Verification items for the finished model (mm, model axes). Coordinates: 2 decimals unless noted, no trailing zeros. Order: outer loops, then holes, each group sorted by start corner. A loop starts at its lowest first (then second) coordinate and runs counter-clockwise, first axis right, second up. Notation, with made-up numbers: (68.5, -34) -> (96.5, -34) arc R33 ccw to (96.5, 1) -> close; hole circle Ø11 at (69, 88). An arc over 180 degrees is marked (long way). Write item = value, one per line. Start each with the question number.
1. Cross-section at C-C on x = 13.5. Record the cut outline in (y, z), plus the area to 3 significant figures.
2. Thickness scan on line 1 along Z through (x, y) = (5.5, 20.5); line 2 along X through (y, z) = (21.25, -4); line 3 along Z through (x, y) = (-8.5, 21.5). Record the ranges inside material, lowest first. Write a range as from..to.
3. Cross-section at A-A on y = 23. Record the cut outline in (x, z), plus the area to 3 significant figures.
4. Go/stop test with flat-tipped pins: P1, Ø4, axis at x = 8.5, z = 1, coming from the -Y side; P2, Ø8, axis at x = 2.5, z = -8, coming from the -Y side; P3, Ø3, axis at x = -12, z = 6, coming from the +Y side. Record where each tip stops, or that it passes through.
5. Cross-section at B-B on z = -2. Record the cut outline in (x, y).
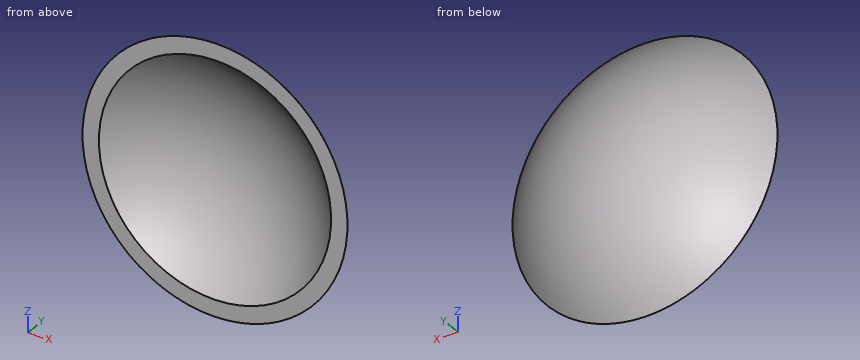
from build123d import *

# Parameters (mm, degrees)
BOX_W           = 60
BOX_H           = 60
BOX_DEPTH       = 60
SPHERE001_ANGLE = 180
SPHERE_ANGLE    = 180


with BuildPart() as cube:
    # Box → Box (new body)
    with BuildSketch(Plane(origin=(-30, -40, -30), x_dir=(1, 0, 0), z_dir=(0, 0, 1))):
        with Locations((30, 30)):
            Rectangle(BOX_W, BOX_H)
    extrude(amount=BOX_DEPTH)


with BuildPart() as inner:
    # Sphere001 → Sphere001 (revolve)
    with BuildSketch(Plane.XZ):
        with BuildLine():
            ThreePointArc((0, -28), (28, 0), (0, 28))
            Line((0, 28), (0, -28))
        make_face()
    revolve(axis=Axis((0, 0, 0), (0, 0, 1)), revolution_arc=SPHERE001_ANGLE)


with BuildPart() as cutshell:
    # Sphere → Sphere (revolve)
    with BuildSketch(Plane.XZ):
        with BuildLine():
            ThreePointArc((0, -30), (30, 0), (0, 30))
            Line((0, 30), (0, -30))
        make_face()
    revolve(axis=Axis((0, 0, 0), (0, 0, 1)), revolution_arc=SPHERE_ANGLE)

    # Cut: cut Inner
    add(inner.part, mode=Mode.SUBTRACT)

    # Cut001: cut Cube
    add(cube.part, mode=Mode.SUBTRACT)


solid = cutshell.part
Worked out:
q1.outline = (20, -17.83) arc R26.79 ccw to (20, 17.83) -> (20, 14.2) arc R24.53 cw to (20, -14.2) -> close
q1.area = 78.5 mm²
q2.line_1 = -21.2..-18.26, 18.26..21.2
q2.line_2 = -20.8..-17.79, 17.79..20.8
q2.line_3 = -19.12..-15.8, 15.8..19.12
q3.outline = circle Ø38.52 at (0, 0); hole circle Ø31.94 at (0, 0)
q3.area = 364 mm²
q4.P1 = 25.93
q4.P2 = 25.11
q4.P3 = 27.53
q5.outline = (-22.27, 20) -> (-19.49, 20) arc R27.93 cw to (19.49, 20) -> (22.27, 20) arc R29.93 ccw to start
